Geometry: final body of the model. Coordinates: model frame, mm. A direction names the side the tool comes from. Give positions to 0.01 mm unless a question says otherwise; leave off trailing zeros. Loops run counter-clockwise (first coordinate to the right, second up) from the corner with the lowest first, then second, coordinate; pieces in that order, holes last. Notation, with made-up numbers: (25, -20) - (62, -20) arc R27 cw to (62, 9) - close; hole circle Ø2 at (57, 34). An arc over 180 degrees is marked (long way). Use one line per item in the form item = value.
```python
from build123d import *

# Parameters (mm, degrees)
SKETCH5_W           = 30
SKETCH5_H           = 25
BOSS_EXTRUDE2_DEPTH = 25
CUT_EXTRUDE2_DEPTH  = 30
SKETCH7_W           = 5
SKETCH7_H           = 15
CUT_EXTRUDE3_DEPTH  = 10
CUT_EXTRUDE4_DEPTH  = 5
SKETCH12_W          = 10
SKETCH12_H          = 10
CUT_EXTRUDE7_DEPTH  = 10
CUT_EXTRUDE8_DEPTH  = 10
CUT_EXTRUDE9_DEPTH  = 20
CUT_EXTRUDE12_DEPTH = 5


with BuildPart() as part:
    # Sketch5 → Boss-Extrude2 (new body)
    with BuildSketch(Plane.XY):
        with Locations((15, 12.5)):
            Rectangle(SKETCH5_W, SKETCH5_H)
    extrude(amount=BOSS_EXTRUDE2_DEPTH)

    # Sketch6 → Cut-Extrude2 (cut)
    with BuildSketch(Plane.ZY):
        Polygon((25, 25), (25, 5), (5, 25), align=None)
    extrude(amount=-CUT_EXTRUDE2_DEPTH, mode=Mode.SUBTRACT)

    # Sketch7 → Cut-Extrude3 (cut)
    with BuildSketch(Plane.ZY):
        with Locations((2.5, 7.5)):
            Rectangle(SKETCH7_W, SKETCH7_H)
    extrude(amount=-CUT_EXTRUDE3_DEPTH, mode=Mode.SUBTRACT)

    # Sketch9 → Cut-Extrude4 (cut)
    with BuildSketch(Plane(origin=(0, 0, 0), x_dir=(-1, 0, 0), z_dir=(0, -1, 0))):
        Polygon((0, -25), (0, -5), (-10, -5), align=None)
    extrude(amount=-CUT_EXTRUDE4_DEPTH, mode=Mode.SUBTRACT)

    # Sketch12 → Cut-Extrude7 (cut)
    with BuildSketch(Plane(origin=(0, 25, 0), x_dir=(1, 0, 0), z_dir=(0, 1, 0))):
        with Locations((25, -5)):
            Rectangle(SKETCH12_W, SKETCH12_H)
    extrude(amount=-CUT_EXTRUDE7_DEPTH, mode=Mode.SUBTRACT)

    # Sketch13 → Cut-Extrude8 (cut)
    with BuildSketch(Plane(origin=(30, 0, 0), x_dir=(0, 0, -1), z_dir=(1, 0, 0))):
        Polygon((-10, 15), (-15, 15), (-10, 20), align=None)
    extrude(amount=-CUT_EXTRUDE8_DEPTH, mode=Mode.SUBTRACT)

    # Sketch14 → Cut-Extrude9 (cut)
    with BuildSketch(Plane(origin=(0, 0, 0), x_dir=(-1, 0, 0), z_dir=(0, 0, -1))):
        Polygon((0, 25), (-10, 25), (0, 15), align=None)
    extrude(amount=-CUT_EXTRUDE9_DEPTH, mode=Mode.SUBTRACT)

    # Sketch15 → Cut-Extrude12 (cut)
    with BuildSketch(Plane(origin=(0, 0, 0), x_dir=(-1, 0, 0), z_dir=(0, -1, 0))):
        Polygon((-30, 0), (-30, -25), (-10, -25), align=None)
    extrude(amount=-CUT_EXTRUDE12_DEPTH, mode=Mode.SUBTRACT)


solid = part.part
```
(1) Cut plane A-A (z = 23.5). Return the cut outline in (x, y), plus the area to 4 significant figures.
Solution:
outline = (0, 5) - (0.75, 5) - (0.75, 0) - (11.2, 0) - (11.2, 5) - (30, 5) - (30, 6.5) - (0, 6.5) - close
area = 97.25 mm2
(2) Cut plane B-B (x = 5.25). Return the cut outline in (y, z).
Solution:
outline = (0, 14.5) - (5, 14.5) - (5, 5) - (15, 5) - (15, 0) - (20.25, 0) - (20.25, 9.75) - (5, 25) - (0, 25) - close
(3) Pin query (flat end, axial travel): P1, Ø11, axis at y = 19.5, z = 6, coming from the +X side; P2, Ø5, axis at x = 4.5, y = 15, coming from the +Z side; P3, Ø4, axis at y = 5, z = 2, coming from the -X side; P4, Ø2, axis at x = 22.5, z = 20.5, coming from the -Y side. Return the tip coordinate at first contact, or that it passes through.
Solution:
P1 = 30
P2 = 17.5
P3 = 10
P4 = 5
(4) Access query for faces 1 (the face through (20, 19, 6)), 2 (the face through (5, 2, 15)), 3 (the face through (25, 5, 18)). Directions: +Z, -Z, +X, -X, +Y, -Y. A direction counts if a zero-diameter tool reaches every point of the face in a straight line with its end or side. Return the directions, or none.
Solution:
face_1 = +Z, -Z, +X, +Y
face_2 = -Z, -X, -Y
face_3 = +Z, +X, -Y
(5) Cut plane D-D (z = 16.5). Return the cut outline in (x, y).
Solution:
outline = (0, 5) - (4.25, 5) - (4.25, 0) - (16.8, 0) - (16.8, 5) - (30, 5) - (30, 13.5) - (0, 13.5) - close
(6) Cut plane C-C (y = 12.75). Return the cut outline in (x, z).
Solution:
outline = (0, 5) - (10, 5) - (10, 0) - (30, 0) - (30, 17.25) - (0, 17.25) - close
(7) Material intervals for L1, parallel to Y at x = 23.25, z = 10.5; L2, parallel to X at y = 8.25, z = 4; L3, parallel to Z at x = 18, y = 3, sorted ascending. Write a range as from..to.
Solution:
L1 = 5..15
L2 = 10..30
L3 = 0..15
